```python
from build123d import *

# Parameters (mm, degrees)
EXTRUDE_1_DEPTH     = 3
SKETCH_2_R          = 1.5
CUT_EXTRUDE_1_DEPTH = 3


with BuildPart() as part:
    # 草图1 → 凸台-拉伸1 (new body)
    with BuildSketch(Plane.XY):
        with BuildLine():
            Line((-31.324082862, 0), (40.675917138, 0))
            ThreePointArc((40.675917138, 0), (42.090130701, -0.585786438), (42.675917138, -2))
            Line((42.675917138, -2), (42.675917138, -34))
            ThreePointArc((42.675917138, -34), (42.090130701, -35.414213562), (40.675917138, -36))
            Line((40.675917138, -36), (-31.324082862, -36))
            ThreePointArc((-31.324082862, -36), (-32.738296424, -35.414213562), (-33.324082862, -34))
            Line((-33.324082862, -34), (-33.324082862, -2))
            ThreePointArc((-33.324082862, -2), (-32.738296424, -0.585786438), (-31.324082862, 0))
        make_face()
    extrude(amount=EXTRUDE_1_DEPTH)

    # 草图2 → 切除-拉伸1 (cut)
    with BuildSketch(Plane.XY.offset(3)):
        with Locations((-24.624082862, -18)):
            Circle(SKETCH_2_R)
        with Locations((33.975917138, -18)):
            Circle(SKETCH_2_R)
        with Locations((-25.062556893, -6.477)):
            Circle(SKETCH_2_R)
        with Locations((33.992443107, -5.08)):
            Circle(SKETCH_2_R)
        with Locations((33.992443107, -9.08)):
            Circle(SKETCH_2_R)
    extrude(amount=-CUT_EXTRUDE_1_DEPTH, mode=Mode.SUBTRACT)


solid = part.part
```
Model file for the job. Use its own axes, mm. Round coordinates to 2 decimals unless told otherwise and drop trailing zeros. Loops run counter-clockwise (first coordinate to the right, second up) from the corner with the lowest first, then second, coordinate; pieces in that order, holes last. Notation, with made-up numbers: M 81.25,2.25 L 99.25,2.25 A15 ccw 99.25,20.25 Z; hole C -38,13 d5. An arc over 180 degrees is marked long. Put each result on its own line as item: value. Start each with the question number.
Item 1: Drop a flat-ended pin along its axis: P1, Ø1.8, axis at x = 33.99, y = -5.08, coming from the +Z side. Give the stop position or say it passes through.
Item 2: Cut at B-B (y = -18). List the corners of the cut face in (x, z).
Item 3: Drill centre lines: line 1 along X through (y, z) = (-17, 0.3); line 2 along X through (y, z) = (-9.5, 2.75). Where is each one in solid material? Low to high.
Item 4: Cut at A-A (y = -9.08). List the corners of the cut face in (x, z).
Item 5: Mould opens along Y. For faces 1 (the face through (42.676, -18, 1)), 2 (the face through (42.106, -35.399, 1.479)), 3 (the face through (4, 0, 1)), 4 (the face through (-26.56, -6.41, 1.52)) say: released by +Y, released by -Y, zero draft, split by the parting line, or undercut.
Answer block:
1. P1: through
2. outline: M -33.32,0 L -26.12,0 L -26.12,3 L -33.32,3 Z; M -23.12,0 L 32.48,0 L 32.48,3 L -23.12,3 Z; M 35.48,0 L 42.68,0 L 42.68,3 L 35.48,3 Z
3. line 1: -33.32 to -25.74, -23.51 to 32.86, 35.09 to 42.68
3. line 2: -33.32 to 32.55, 35.43 to 42.68
4. outline: M -33.32,0 L 32.49,0 L 32.49,3 L -33.32,3 Z; M 35.49,0 L 42.68,0 L 42.68,3 L 35.49,3 Z
5. face 1: zero draft
5. face 2: released by -Y
5. face 3: released by +Y
5. face 4: undercut
